Source: CAD feature listing. Evaluate the final solid. Frame: model axes, mm. Face numbers are marked on the shaded views. A direction names the side the tool comes from. Give positions to 0.01 mm unless a question says otherwise; leave off trailing zeros. Write each loop counter-clockwise with the first axis right and the second up, starting at its lowest first coordinate (ties: lowest second). Pieces come first, ordered by that corner, then holes. Notation, with made-up numbers: (-4.5, 50.5) -> (28.5, 50.5) arc R37 cw to (28.5, 87.5) -> close; hole circle Ø2 at (72.25, -9.75). An arc over 180 degrees is marked (long way). Write item = value, one per line.
Autodesk Fusion 360 part; units mm, degrees
sketch "Sketch1" plane through (0, 0, 0) normal (1, 0, 0) x (0, 1, 0)
  line L0 (5.5, 2.25) -> (-5.5, 2.25)
  line L1 (-6, 1.75) -> (-6, -1.75)
  line L2 (-5.5, -2.25) -> (5.5, -2.25)
  line L3 (6, -1.75) -> (6, 1.75)
  line L4 (6, 2.25) -> (-6, -2.25) construction
  line L5 (-6, 2.25) -> (6, -2.25) construction
  arc A0 (-5.5, 2.25) -> (-6, 1.75) centre (-5.5, 1.75) ccw
  arc A1 (-6, -1.75) -> (-5.5, -2.25) centre (-5.5, -1.75) ccw
  arc A2 (6, 1.75) -> (5.5, 2.25) centre (5.5, 1.75) ccw
  arc A3 (5.5, -2.25) -> (6, -1.75) centre (5.5, -1.75) ccw
  dimension "d1" = 12
  dimension "d2" = 4.5
  dimension "d3" = 0.5
  dimension "d4" = 0.5
  dimension "d5" = 0.5
  dimension "d6" = 0.5
extrude "Extrude1" add sketch "Sketch1" along normal blind 18.8
sketch "Sketch2" plane through (18.8, 0, 0) normal (1, 0, 0) x (0, 1, 0)
  arc A0 (5.5, -2.25) -> (6, -1.75) centre (5.5, -1.75) ccw
  line L0 (6, -1.75) -> (6, 1.75)
  arc A1 (6, 1.75) -> (5.5, 2.25) centre (5.5, 1.75) ccw
  line L1 (5.5, 2.25) -> (-5.5, 2.25)
  arc A2 (-5.5, 2.25) -> (-6, 1.75) centre (-5.5, 1.75) ccw
  line L2 (-6, 1.75) -> (-6, -1.75)
  arc A3 (-6, -1.75) -> (-5.5, -2.25) centre (-5.5, -1.75) ccw
  line L3 (-5.5, -2.25) -> (5.5, -2.25)
  line L4 (0, 2.25) -> (0, -0.75)
  line L5 (0, -0.75) -> (6, -0.75)
  line L6 (6, -0.75) -> (6, -2.25)
  line L7 (6, -2.25) -> (0, -2.25)
  line L8 (0, -2.25) -> (0, -0.75)
  line L9 (0, -0.75) -> (-6, -0.75)
  line L10 (-6, -0.75) -> (-6, -2.25)
  line L11 (-6, -2.25) -> (0, -2.25)
  line L12 (0, -2.25) -> (0, -0.75)
  dimension "d9" = 3
extrude "Extrude2" cut sketch "Sketch2" against normal blind 4 contours A0 L0 L3 L5 L6 L7 L8 L12 | L2 A3 L3 L8 L9 L10 L11 L12
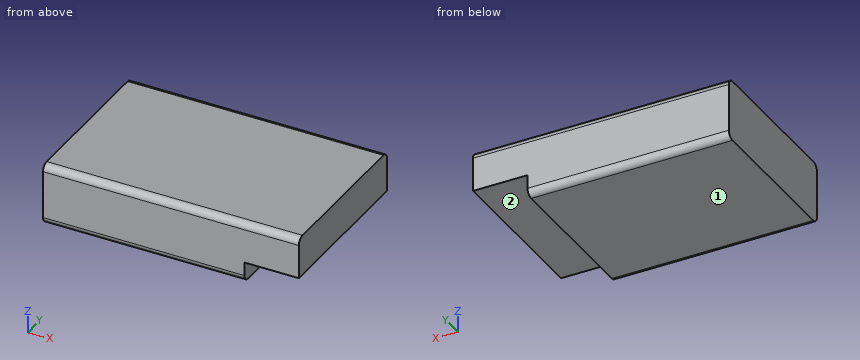
(1) Section query B-B (x = 17.5). Return loops of the section in (y, z).
Values follow:
outline = (-6, -0.75) -> (6, -0.75) -> (6, 1.75) arc R0.5 ccw to (5.5, 2.25) -> (-5.5, 2.25) arc R0.5 ccw to (-6, 1.75) -> close
(2) First-contact query: pin 1 (4.5 mm diameter, centred on x = 17.5, y = 0, fed in from -Z). Flat tip, straight axial feed; report the tip coordinate or a pass-through.
Values follow:
pin_1 = -0.75
(3) Section query C-C (z = -1.5). Return loops of the section in (x, y).
Values follow:
outline = (0, -6) -> (14.8, -6) -> (14.8, 6) -> (0, 6) -> close
(4) Section query A-A (y = -4.75). Return loops of the section in (x, z).
Values follow:
outline = (0, -2.25) -> (14.8, -2.25) -> (14.8, -0.75) -> (18.8, -0.75) -> (18.8, 2.25) -> (0, 2.25) -> close
(5) Access query for the marked faces 1 and 2. Directions: +Z, -Z, +X, -X, +Y, -Y. A direction counts if a zero-diameter tool reaches every point of the face in a straight line with its end or side. Return the directions, or none.
Values follow:
face_1 = -Z, +X, -X, +Y, -Y
face_2 = -Z, +X, +Y, -Y
(6) Material intervals for line 1 (X direction, y = 5.25, z = -1.7); line 2 (Z direction, x = 16.5, y = -3.5), sorted ascending.
Values follow:
line_1 = 0 to 14.8
line_2 = -0.75 to 2.25
